from build123d import *

# Parameters (mm, degrees)
SKETCH1_W                        = 25.4
SKETCH1_H                        = 25.4
BOSS_EXTRUDE1_DEPTH              = 69.341499747
F_6_05_6_05_DIAMETER_HOLE1_D     = 6.05
TAP_DRILL_FOR_M6X0_75_TAP1_D     = 5.25
TAP_DRILL_FOR_M6X0_75_TAP1_DEPTH = 14.732


with BuildPart() as part:
    # Sketch1 → Boss-Extrude1 (new body, symmetric)
    with BuildSketch(Plane.XY):
        Rectangle(SKETCH1_W, SKETCH1_H)
    extrude(amount=BOSS_EXTRUDE1_DEPTH, both=True)

    # Ø6.05 (6.05) Diameter Hole1 (through all)
    with Locations(Plane(origin=(0, -12.7, 0), x_dir=(-1, 0, 0), z_dir=(0, -1, 0))):
        with Locations((0, -5.841499747), (0, -56.641499747)):
            Hole(F_6_05_6_05_DIAMETER_HOLE1_D / 2)

    # Tap Drill for M6x0.75 Tap1
    with Locations(Plane(origin=(0, 0, -69.341499747), x_dir=(-1, 0, 0), z_dir=(0, 0, -1))):
        with Locations((0, 0)):
            Hole(TAP_DRILL_FOR_M6X0_75_TAP1_D / 2, depth=TAP_DRILL_FOR_M6X0_75_TAP1_DEPTH)


solid = part.part
Can you work these out from the model? Positions are in its coordinate system, mm. A direction names the side the tool comes from. Round coordinates to 2 decimals unless told otherwise and drop trailing zeros. Loops run counter-clockwise (first coordinate to the right, second up) from the corner with the lowest first, then second, coordinate; pieces in that order, holes last. Notation, with made-up numbers: (-19, -4.75) - (32, -4.75) arc R10 cw to (32, 5.25) - close; hole circle Ø2 at (-27.75, 45.25). An arc over 180 degrees is marked (long way). Use CSV: the item, a comma, the result in double quotes. Start each with the question number.
1) We'd pull the mould along Y, two halves only. Please class faces 3 (the flat face through (0, -12.7, 1)), 4 (the flat face through (12.7, 0, 1)), 5 (the cylindrical face through (2.5, 0.8, -61.9)): released by +Y, released by -Y, zero draft, split by the parting line, or undercut.
2) For faces 1 (the flat face through (3, 0, -69.341)), 2 (the flat face through (0, 0, -54.609)), which set-ups out of +Z, -Z, +X, -X, +Y, -Y let a thin tool reach every point of the face, with its end or its side?
3) If we section it at A-A on x = 0: Write out the boundary of the cut face in (y, z) (1 decimal).
4) Please list where these lines run through material, in increasing order: probe 1 along Z at (x, y) = (0, -6.75); probe 2 along Y at (x, z) = (0, -59) (3 decimals); probe 3 along Z at (x, y) = (-0.75, 2.75). Write a range as [from, to].
5) If we section it at B-B on y = 0: Count the separate pieces of the cut face and the enclosed holes in it, plus the area to 3 significant figures.
Geometry results:
1,face 3,"released by -Y"
1,face 4,"zero draft"
1,face 5,"undercut"
2,face 1,"-Z, +X, -X, +Y, -Y"
2,face 2,"-Z"
3,outline,"(-12.7, -69.3) - (-2.6, -69.3) - (-2.6, -54.6) - (2.6, -54.6) - (2.6, -69.3) - (12.7, -69.3) - (12.7, 2.8) - (-12.7, 2.8) - close; (-12.7, 8.9) - (12.7, 8.9) - (12.7, 53.6) - (-12.7, 53.6) - close; (-12.7, 59.7) - (12.7, 59.7) - (12.7, 69.3) - (-12.7, 69.3) - close"
4,probe 1,"z = [-69.34, 2.82], [8.87, 53.62], [59.67, 69.34]"
4,probe 2,"y = [-12.7, -2.625], [2.625, 12.7]"
4,probe 3,"z = [-69.34, 2.91], [8.77, 53.71], [59.57, 69.34]"
5,separate pieces,"1"
5,enclosed holes,"2"
5,area,"3,390 mm2"
